CAD build for the part. Positions are in the model's coordinates, mm. Face numbers are marked on the shaded views. A direction names the side the tool comes from. Coordinates: 2 decimals unless noted, no trailing zeros. Loops run counter-clockwise (first coordinate to the right, second up) from the corner with the lowest first, then second, coordinate; pieces in that order, holes last. Notation, with made-up numbers: (-26.5, 10.25) -> (18.5, 10.25) arc R36 ccw to (18.5, 45.25) -> close; hole circle Ø8 at (39, 62.5). An arc over 180 degrees is marked (long way). Write each question's results on one line, items separated by ' | '.
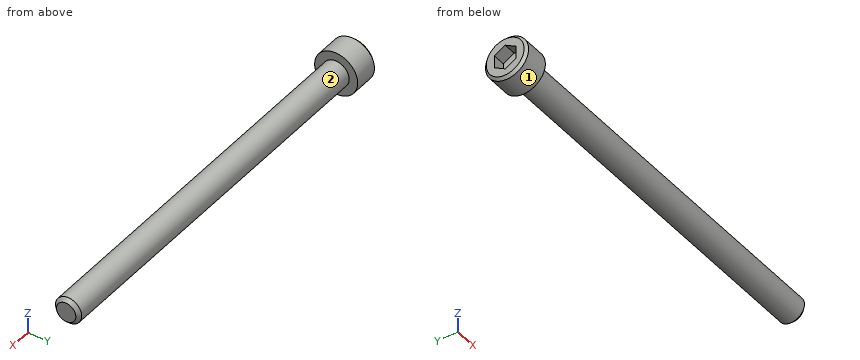
from build123d import *

# Parameters (mm, degrees)
HEXDRIVE_DEPTH = 2.286


with BuildPart() as part:
    # BodySketch → BaseBody (revolve)
    with BuildSketch(Plane(origin=(0, 0, 0), x_dir=(1, 0, 0), z_dir=(0, 1, 0)), mode=Mode.PRIVATE) as basebody_sk:
        Polygon((0, 2.413), (0, 3.96875), (-4.3434, 3.96875), (-4.826, 3.48615), (-4.826, 0), (69.85, 0), (69.85, 1.78308), (69.22008, 2.413), align=None)
    revolve(basebody_sk.sketch.rotate(Axis((-4.826, 0, 0), (1, 0, 0)), 180), axis=Axis((-4.826, 0, 0), (1, 0, 0)))

    # DriveSketch → HexDrive (cut)
    with BuildSketch(Plane.ZY.offset(4.826)):
        Polygon((2.292092116, 0), (1.146046058, 1.98501), (-1.146046058, 1.98501), (-2.292092116, 0), (-1.146046058, -1.98501), (1.146046058, -1.98501), align=None)
    extrude(amount=-HEXDRIVE_DEPTH, mode=Mode.SUBTRACT)


solid = part.part
1) Slice it at A-A (z = 0). Write the cut outline in (x, y), then the cut area to 3 significant figures.
Outcome:
outline: (-4.83, -3.49) -> (-4.34, -3.97) -> (0, -3.97) -> (0, -2.41) -> (69.22, -2.41) -> (69.85, -1.78) -> (69.85, 1.78) -> (69.22, 2.41) -> (0, 2.41) -> (0, 3.97) -> (-4.34, 3.97) -> (-4.83, 3.49) -> (-4.83, 1.99) -> (-2.54, 1.99) -> (-2.54, -1.99) -> (-4.83, -1.99) -> close | area: 366 mm^2
2) Drill centre lines: L1, parallel to Y at x = 65.5, z = 0.75; L2, parallel to X at y = 1, z = -1.25. Where is each one in solid material? Low to high. Write a range as from..to.
Outcome:
L1: y = -2.29..2.29 | L2: x = -2.54..69.85
3) Which spindle directions (+Z, -Z, +X, -X, +Y, -Y) get a long thin tool onto all of the face, cutting with end or side? Do the marked faces 1 and 2. Say none if no direction does.
Outcome:
face 1: +X, -X | face 2: +X
4) Pin check, flat tips, straight feed: pin 1 (1 mm diameter, centred on x = 21.5, z = 1.5, fed in from -Y); pin 2 (4.5 mm diameter, centred on y = 1, z = 0, fed in from -X); pin 3 (1.5 mm diameter, centred on x = 15, y = -2.5, fed in from +Z); pin 4 (0.7 mm diameter, centred on x = -3.5, z = 0.5, fed in from -Y). Stop position of each tip, or through.
Outcome:
pin 1: stops at y = -2.2 | pin 2: stops at x = -4.83 | pin 3: stops at z = 1.66 | pin 4: stops at y = -3.97
5) Slice it at B-B (x = 23.5). Write the cut outline in (y, z).
Outcome:
outline: circle Ø4.83 at (0, 0)
